Design review of the part built by this model. Coordinates are the model's own, in mm. A direction names the side the tool comes from. Round coordinates to 2 decimals unless told otherwise and drop trailing zeros. Loops run counter-clockwise (first coordinate to the right, second up) from the corner with the lowest first, then second, coordinate; pieces in that order, holes last. Notation, with made-up numbers: (57, 6) - (80, 6) arc R24 cw to (80, 30) - close; hole circle Ø2 at (-9, 24). An arc over 180 degrees is marked (long way). Use one line per item in the form item = value. Start each with the question number.
(1) We need section B-B, the plane x = 1.75. Write out the cut boundary in (y, z), then the cut area to 3 significant figures.
(2) We need section C-C, the plane z = 13.5. Write out the cut boundary in (x, y), then the cut area to 3 significant figures.
(3) We need section D-D, the plane y = 8.75. Write out the cut boundary in (x, z), then the cut area to 3 significant figures.
(4) Wall thickness on probe 1 along Z at (x, y) = (1.75, 8.5); probe 2 along X at (y, z) = (-0.5, 78.5); probe 3 along Y at (x, z) = (-0.25, 70.5): over which ranges is each line inside the solid? List them lowest first. Write a range as [from, to].
(5) For pin 1 (3 mm diameter, centred on x = 0.5, z = 15.5, fed in from -Y); pin 2 (1.5 mm diameter, centred on x = 1.5, y = -8.5, fed in from +Z); pin 3 (6 mm diameter, centred on x = -5, z = 78.5, fed in from +Y), all flat-tipped, find the tip position at first contact; note any pin that passes through.
(6) Machinability: for faces 1 (the cylindrical face through (-1.38, 6.2, 43.83)), 2 (the flat face through (9.525, 0, -6)), which of the approach directions +Z, -Z, +X, -X, +Y, -Y give a long, thin tool a straight path to every point of the face, cutting with its end or side? Answer none if there is none.
(7) We need section A-A, the plane y = 0. Write out the cut boundary in (x, z) (3 decimals).
Autodesk Inventor part; units mm, degrees
ref_plane "YZ Plane" through (0, 0, 0) normal (1, 0, 0) x (0, 1, 0)
ref_plane "XZ Plane" through (0, 0, 0) normal (0, 1, 0) x (-1, 0, 0)
ref_plane "XY Plane" through (0, 0, 0) normal (0, 0, 1) x (1, 0, 0)
sketch "Sketch1" plane through (0, 0, 0) normal (0, 0, 1) x (1, 0, 0)
  circle A0 centre (0, 0) radius 6.35
  line L0 (0, 10.9985) -> (9.525, 5.4993)
  line L1 (9.525, 5.4993) -> (9.525, -5.4993)
  line L2 (9.525, -5.4993) -> (0, -10.9985)
  line L3 (0, -10.9985) -> (-9.525, -5.4993)
  line L4 (-9.525, -5.4993) -> (-9.525, 5.4993)
  line L5 (-9.525, 5.4993) -> (0, 10.9985)
  dimension "d1" = 19.05
extrude "Extrusion1" add sketch "Sketch1" against normal blind 12.7 contours A0 | L0 L1 L2 L3 L4 L5
sketch "Sketch2" plane through (0, 0, 0) normal (0, 0, 1) x (1, 0, 0)
  circle A0 centre (0, 0) radius 6.35
  dimension "d4" = 12.7
extrude "Extrusion2" add sketch "Sketch2" along normal blind 88.9
thread "Thread1"
properties part number "4 in bolt"
Data:
q1.outline = (-9.99, -12.7) - (9.99, -12.7) - (9.99, 0) - (6.1, 0) - (6.1, 88.9) - (-6.1, 88.9) - (-6.1, 0) - (-9.99, 0) - close
q1.area = 1,340 mm^2
q2.outline = circle Ø12.7 at (0, 0)
q2.area = 127 mm^2
q3.outline = (-3.89, -12.7) - (3.89, -12.7) - (3.89, 0) - (-3.89, 0) - close
q3.area = 98.9 mm^2
q4.probe_1 = [-12.7, 0]
q4.probe_2 = [-6.33, 6.33]
q4.probe_3 = [-6.35, 6.35]
q5.pin_1 = -6.35
q5.pin_2 = 0
q5.pin_3 = 6.03
q6.face_1 = +Z
q6.face_2 = +Z, -Z, +X, +Y, -Y
q7.outline = (-9.525, -12.7) - (9.525, -12.7) - (9.525, 0) - (6.35, 0) - (6.35, 88.9) - (-6.35, 88.9) - (-6.35, 0) - (-9.525, 0) - close
